Could you check a few things on this drawing? It's one solid part, dimensions in mm from its lowest x, y, z. A direction names the side the tool comes from. Give positions to 0.01 mm unless a question says otherwise; leave off trailing zeros. Loops run counter-clockwise (first coordinate to the right, second up) from the corner with the lowest first, then second, coordinate; pieces in that order, holes last. Notation, with made-up numbers: M 11,22 L 35,22 A16 ccw 35,39 Z; hole C 74.25,34.5 d11. An arc over 180 degrees is marked long. Answer as a JSON object with one key per item and string values.
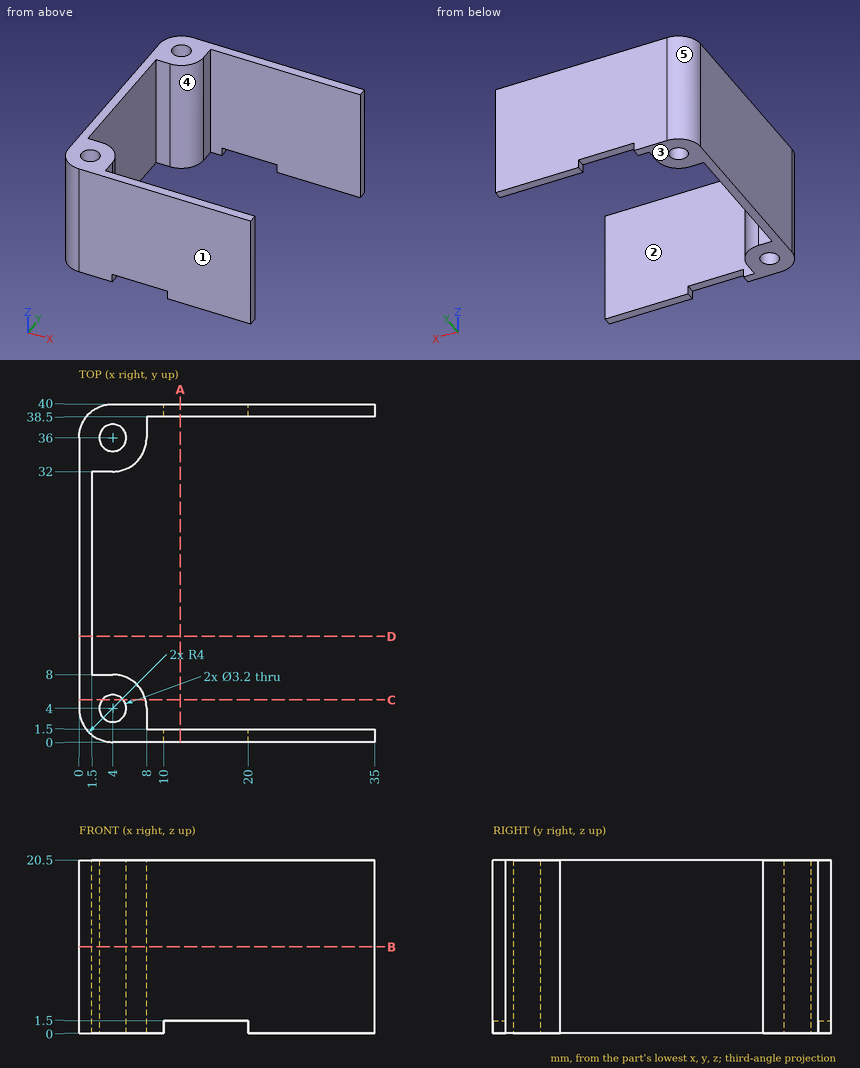
1) Please list where these lines run through material, in increasing order: line 1 along Y through (x, z) = (10, 2); line 2 along X through (y, z) = (16, 13); line 3 along Y through (x, z) = (6, 10.75). Write a range as from..to.
Answer list:
{"line 1": "0..1.5, 38.5..40", "line 2": "0..1.5", "line 3": "0..7.46, 32.54..40"}
2) If we mould it in two halves opening along Y, with no side actions, what happens to the marked faces 1, 2 and 3? For each: +Y half, -Y half, draft (parallel to the pull), parting line (faces both ways), or undercut.
Answer list:
{"face 1": "-Y half", "face 2": "undercut", "face 3": "draft"}
3) Suppose I cut it at C-C, the plane y = 5. Write out the boundary of the cut face in (x, z).
Answer list:
{"outline": "M 0,0 L 2.75,0 L 2.75,20.5 L 0,20.5 Z; M 5.25,0 L 7.87,0 L 7.87,20.5 L 5.25,20.5 Z"}
4) Suppose I cut it at A-A, the plane x = 12. Write out the boundary of the cut face in (y, z), and give its area (3 significant figures).
Answer list:
{"outline": "M 0,1.5 L 1.5,1.5 L 1.5,20.5 L 0,20.5 Z; M 38.5,1.5 L 40,1.5 L 40,20.5 L 38.5,20.5 Z", "area": "57.0 mm^2"}
5) Suppose I cut it at D-D, the plane y = 12.5. Write out the boundary of the cut face in (x, z).
Answer list:
{"outline": "M 0,0 L 1.5,0 L 1.5,20.5 L 0,20.5 Z"}
6) Will these pins go through, and if not, where does the flat tip stop? pin 1 Ø10 at (y, z) = (21.5, 10) entering from +X; pin 2 Ø1.2 at (y, z) = (37, 5.5) entering from +X; pin 3 Ø1.2 at (x, y) = (17.5, 39) entering from -Z.
Answer list:
{"pin 1": "x = 1.5", "pin 2": "x = 8", "pin 3": "z = 1.5"}
7) Suppose I cut it at B-B, the plane z = 10.25. Write out the boundary of the cut face in (x, y), and give its area (3 significant figures).
Answer list:
{"outline": "M 0,4 A4 ccw 4,0 L 35,0 L 35,1.5 L 8,1.5 L 8,4 A4 ccw 4,8 L 1.5,8 L 1.5,32 L 4,32 A4 ccw 8,36 L 8,38.5 L 35,38.5 L 35,40 L 4,40 A4 ccw 0,36 Z; hole C 4,4 d3.2; hole C 4,36 d3.2", "area": "215 mm^2"}
8) For the marked faces 4 and 5, which set-ups out of +Z, -Z, +X, -X, +Y, -Y let a thin tool reach every point of the face, with its end or its side?
Answer list:
{"face 4": "+Z, -Z, +X", "face 5": "+Z, -Z, -X, +Y"}
